Source: CAD feature listing. Evaluate the final solid. Frame: model axes, mm. Face numbers are marked on the shaded views. A direction names the side the tool comes from. Give positions to 0.01 mm unless a question says otherwise; leave off trailing zeros. Order: outer loops, then holes, each group sorted by start corner. A loop starts at its lowest first (then second) coordinate and runs counter-clockwise, first axis right, second up.
```python
from build123d import *

# Parameters (mm, degrees)
SKETCH1_R          = 15
EXTRUDE1_DEPTH     = 33
SKETCH2_R          = 7.5
CUT_EXTRUDE1_DEPTH = 3
SKETCH3_R          = 25
EXTRUDE2_DEPTH     = 29.84000001
CUT_EXTRUDE2_DEPTH = 14.732
CIRPATTERN1_COUNT  = 3
SKETCH6_R          = 6.5
CUT_EXTRUDE4_DEPTH = 10
CUT_EXTRUDE3_REACH = 51.637
SKETCH5_R          = 7.8994


with BuildPart() as part:
    # Sketch1 → Extrude1 (new body)
    with BuildSketch(Plane.XY):
        Circle(SKETCH1_R)
    extrude(amount=EXTRUDE1_DEPTH)

    # Sketch2 → Cut-Extrude1 (cut)
    with BuildSketch(Plane(origin=(0, 0, 0), x_dir=(-1, 0, 0), z_dir=(0, 0, -1))):
        Circle(SKETCH2_R)
    extrude(amount=-CUT_EXTRUDE1_DEPTH, mode=Mode.SUBTRACT)

    # Sketch3 → Extrude2 (add)
    with BuildSketch(Plane.XY.offset(4.999999906)):
        Circle(SKETCH3_R)
    extrude(amount=EXTRUDE2_DEPTH)

    # Sketch4 → Cut-Extrude2 (cut)
    with BuildSketch(Plane.XY.offset(34.839999916)):
        Polygon((0, 0), (4.9911, 0), (4.9911, 26.885801132), (-4.9911, 26.885801132), (-4.9911, 0), align=None)
    cut_extrude2 = extrude(amount=-CUT_EXTRUDE2_DEPTH, mode=Mode.SUBTRACT)

    # CirPattern1: Cut-Extrude2 ×3 about axis
    cirpattern1_axis = Axis((0, 0, 0), (0, 0, 1))
    for i in range(1, CIRPATTERN1_COUNT):
        add(cut_extrude2.rotate(cirpattern1_axis, i * 360 / CIRPATTERN1_COUNT), mode=Mode.SUBTRACT)

    # Sketch6 → Cut-Extrude4 (cut)
    with BuildSketch(Plane(origin=(0, 0, 3), x_dir=(-1, 0, 0), z_dir=(0, 0, -1))):
        Circle(SKETCH6_R)
    extrude(amount=-CUT_EXTRUDE4_DEPTH, mode=Mode.SUBTRACT)

    # Cut-Extrude3: up to this face of the body (flat: up to its plane)
    cut_extrude3_end = Plane(part.part.faces().sort_by_distance((0, 0, 13))[0])
    # Sketch5 → Cut-Extrude3 (cut, up to the picked face)
    with BuildSketch(Plane.XY.offset(34.839999916), mode=Mode.PRIVATE) as cut_extrude3_sk1:
        with Locations(Location((0, 0, 0), (0, 0, 9.185472822))):
            Circle(SKETCH5_R)
    cut_extrude3_tool1 = split(extrude(cut_extrude3_sk1.sketch, amount=-CUT_EXTRUDE3_REACH, mode=Mode.PRIVATE), bisect_by=cut_extrude3_end, keep=Keep.BOTH, mode=Mode.PRIVATE)
    add(cut_extrude3_tool1.solids().sort_by(Axis((0, 0, 34.84), (0, 0, -1)))[0], mode=Mode.SUBTRACT)


solid = part.part
```
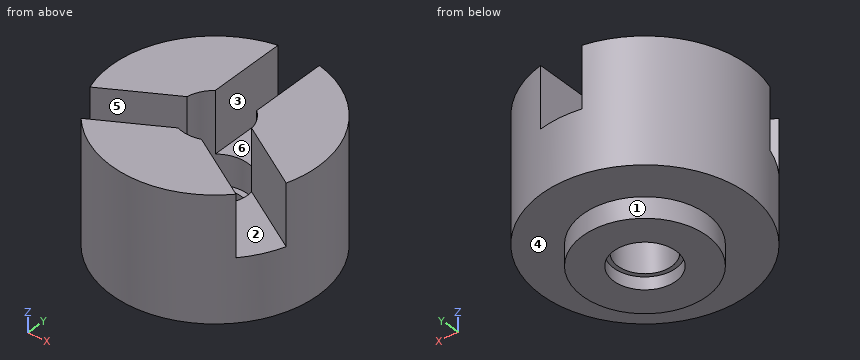
1) Section query A-A, the plane z = 30. Return the cut outline in (x, y).
Report:
outline: (-23.71, -7.93) - (-7.8, 1.26) arc R7.9 cw to (-4.99, 6.12) - (-4.99, 24.5) arc R25 ccw to start; (-18.72, -16.57) arc R25 ccw to (18.72, -16.57) - (2.81, -7.38) arc R7.9 cw to (-2.81, -7.38) - close; (4.99, 6.12) arc R7.9 cw to (7.8, 1.26) - (23.71, -7.93) arc R25 ccw to (4.99, 24.5) - close
2) Reachability of the marked faces 4, 5 and 6 from +Z, -Z, +X, -X, +Y, -Y: full face, straight path, thin tool, end or side. Return the list, or none.
Report:
face 4: -Z
face 5: +Z
face 6: +Z, +Y
3) Material intervals for L1, parallel to Y at x = 0, z = 1.1; L2, parallel to Y at x = 0, z = 9; L3, parallel to Z at x = 17, y = 0.5, sorted ascending.
Report:
L1: y = -15 to -7.5, 7.5 to 15
L2: y = -25 to -6.5, 6.5 to 25
L3: z = 5 to 34.84
4) Section query B-B, the plane x = 0. Return the cut outline in (y, z).
Report:
outline: (-25, 5) - (-15, 5) - (-15, 0) - (-7.5, 0) - (-7.5, 3) - (-6.5, 3) - (-6.5, 13) - (-7.9, 13) - (-7.9, 34.84) - (-25, 34.84) - close; (6.5, 3) - (7.5, 3) - (7.5, 0) - (15, 0) - (15, 5) - (25, 5) - (25, 20.11) - (7.9, 20.11) - (7.9, 13) - (6.5, 13) - close
5) Pin query (flat end, axial travel): pin 1 (3 mm diameter, centred on x = -1, y = 18.5, fed in from +Z); pin 2 (1.5 mm diameter, centred on y = -9.5, z = 28, fed in from +X); pin 3 (6 mm diameter, centred on x = 8, z = 26, fed in from -Y); pin 4 (12 mm diameter, centred on x = 0, y = 0, fed in from +Z). Return the tip coordinate at first contact, or that it passes through.
Report:
pin 1: stops at z = 20.11
pin 2: stops at x = 7.77
pin 3: stops at y = -24.49
pin 4: passes through
6) Section query D-D, the plane z = 6.5. Return the cut outline in (x, y).
Report:
outline: circle Ø50 at (0, 0); hole circle Ø13 at (0, 0)
7) Section query C-C, the plane y = 0. Return the cut outline in (x, z).
Report:
outline: (-25, 5) - (-15, 5) - (-15, 0) - (-7.5, 0) - (-7.5, 3) - (-6.5, 3) - (-6.5, 13) - (-7.9, 13) - (-7.9, 20.11) - (-9.98, 20.11) - (-9.98, 34.84) - (-25, 34.84) - close; (6.5, 3) - (7.5, 3) - (7.5, 0) - (15, 0) - (15, 5) - (25, 5) - (25, 34.84) - (9.98, 34.84) - (9.98, 20.11) - (7.9, 20.11) - (7.9, 13) - (6.5, 13) - close
8) Draft query along Y for the marked faces 1, 2 and 3. Return one class per face: +Y half, -Y half, draft (parallel to the pull), parting line (faces both ways), or undercut.
Report:
face 1: parting line
face 2: undercut
face 3: draft
